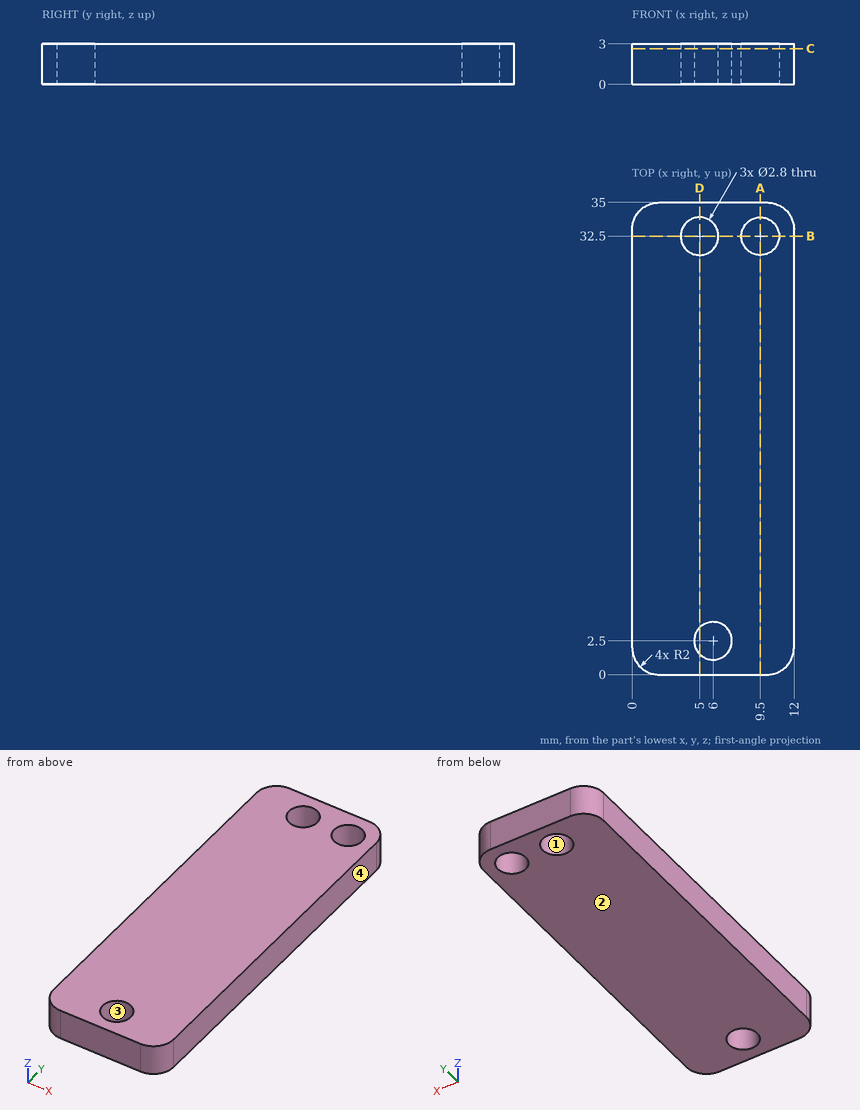
Geometry: see drawing. Coordinates: mm, zero at the bounding-box minimum. Coordinates: 2 decimals unless noted, no trailing zeros. Write each loop counter-clockwise with the first axis right and the second up, starting at its lowest first coordinate (ties: lowest second). Pieces come first, ordered by that corner, then holes.
1) Section C-C on z = 2.65. Output: boundary loops of the cut face in (x, y).
2) Mould query, pull axis X, two halves, no side actions, for the marked faces 1, 2, 3 and 4. Classes: pulls with the +X half, pulls with the -X half, needs draft (parallel to the pull), parting line crosses it, or undercut.
3) Material intervals for line 1 along X through (y, z) = (32.5, 1.9); line 2 along Y through (x, z) = (6, 1.3); line 3 along Y through (x, z) = (9.5, 1.65), sorted ascending.
4) Section A-A on x = 9.5. Output: boundary loops of the cut face in (y, z), and give its area (3 significant figures).
5) Pin query (flat end, axial travel): pin 1 Ø2 at (x, y) = (5, 32.5) entering from +Z. Return the tip coordinate at first contact, or that it passes through.
6) Section D-D on x = 5. Output: boundary loops of the cut face in (y, z), and give its area (3 significant figures).
7) Section B-B on y = 32.5. Output: boundary loops of the cut face in (x, z), and give its area (3 significant figures).
Check result:
1. outline: (0, 2) arc R2 ccw to (2, 0) - (10, 0) arc R2 ccw to (12, 2) - (12, 33) arc R2 ccw to (10, 35) - (2, 35) arc R2 ccw to (0, 33) - close; hole circle Ø2.8 at (5, 32.5); hole circle Ø2.8 at (6, 2.5); hole circle Ø2.8 at (9.5, 32.5)
2. face 1: undercut
2. face 2: needs draft
2. face 3: undercut
2. face 4: pulls with the +X half
3. line 1: x = 0 to 3.6, 6.4 to 8.1, 10.9 to 12
3. line 2: y = 0 to 1.1, 3.9 to 31.52, 33.48 to 35
3. line 3: y = 0 to 31.1, 33.9 to 35
4. outline: (0, 0) - (31.1, 0) - (31.1, 3) - (0, 3) - close; (33.9, 0) - (35, 0) - (35, 3) - (33.9, 3) - close
4. area: 96.6 mm2
5. pin 1: passes through
6. outline: (0, 0) - (1.52, 0) - (1.52, 3) - (0, 3) - close; (3.48, 0) - (31.1, 0) - (31.1, 3) - (3.48, 3) - close; (33.9, 0) - (35, 0) - (35, 3) - (33.9, 3) - close
6. area: 90.7 mm2
7. outline: (0, 0) - (3.6, 0) - (3.6, 3) - (0, 3) - close; (6.4, 0) - (8.1, 0) - (8.1, 3) - (6.4, 3) - close; (10.9, 0) - (12, 0) - (12, 3) - (10.9, 3) - close
7. area: 19.2 mm2
